Here's how the part is built. I have some questions about the finished solid (model axes, mm). Round coordinates to 2 decimals unless told otherwise and drop trailing zeros. Write each loop counter-clockwise with the first axis right and the second up, starting at its lowest first coordinate (ties: lowest second). Pieces come first, ordered by that corner, then holes. Notation, with made-up numbers: (-17, 66) - (28, 66) arc R19 cw to (28, 83) - close; hole circle Ø2 at (1, 6). An arc over 180 degrees is marked (long way). Use one line per item in the form item = value. Start each with the question number.
1. I want a section at B-B, the plane y = -1.75. List the corners of the cut face in (x, z) for me.
2. I want a section at C-C, the plane x = 230. List the corners of the cut face in (y, z) for me.
3. We'd pull the mould along Z, two halves only. Please class faces 1 (the flat face through (116, -4.5, -52)), 2 (the flat face through (-5, -9, 1)), 3 (the flat face through (-344, -4.5, -52)): +Z half, -Z half, draft (parallel to the pull), parting line (faces both ways), or undercut.
4. I want a section at A-A, the plane z = -34.5. List the corners of the cut face in (x, y) for me.
5. I want a section at D-D, the plane z = -68. List the corners of the cut face in (x, y) for me.
6. Will these pins go through, and if not, where does the flat tip stop? pin 1 (2 mm diameter, centred on x = 155.5, y = -1.5, fed in from -Z); pin 2 (2 mm diameter, centred on y = -3, z = 60, fed in from +X); pin 3 (3 mm diameter, centred on y = -2, z = -55.5, fed in from -X).
7. If I drill on line 1 along X through (y, z) = (-7.25, -6); line 2 along X through (y, z) = (-4, -78); line 3 along Z through (x, y) = (-25.5, -0.75), over which ranges is the centre line in solid material (lowest first)?
```python
from build123d import *

# Parameters (mm, degrees)
F0_W      = 740
F0_H      = 200
F1_DEPTH  = 9
F2_W      = 4.5
F2_H      = 200
F3_DEPTH  = 4.5
F4_W      = 4.5
F4_H      = 200
F5_DEPTH  = 4.5
F6_W      = 731
F6_H      = 4.5
F7_DEPTH  = 4.5
F8_W      = 731
F8_H      = 4.5
F9_DEPTH  = 4.5
F10_W     = 150
F10_H     = 95
F11_DEPTH = 25
F12_W     = 4.5
F12_H     = 40.5
F13_DEPTH = 4.5
F14_W     = 4.5
F14_H     = 40.5
F15_DEPTH = 4.5


with BuildPart() as f1:
    # F0 (on Front) → F1 (new body)
    with BuildSketch(Plane.XZ):
        Rectangle(F0_W, F0_H)
    extrude(amount=F1_DEPTH)

    # F2 (on face) → F3 (cut)
    with BuildSketch(Plane.YZ.offset(370)):
        with Locations((-2.25, 0)):
            Rectangle(F2_W, F2_H)
    extrude(amount=-F3_DEPTH, mode=Mode.SUBTRACT)

    # F4 (on face) → F5 (cut)
    with BuildSketch(Plane(origin=(-370, 0, 0), x_dir=(0, -1, 0), z_dir=(-1, 0, 0))):
        with Locations((2.25, 0)):
            Rectangle(F4_W, F4_H)
    extrude(amount=-F5_DEPTH, mode=Mode.SUBTRACT)

    # F6 (on face) → F7 (cut)
    with BuildSketch(Plane(origin=(0, 0, 0), x_dir=(-1, 0, 0), z_dir=(0, 1, 0))):
        with Locations((0, -52.75)):
            Rectangle(F6_W, F6_H)
    extrude(amount=-F7_DEPTH, mode=Mode.SUBTRACT)

    # F8 (on face) → F9 (cut)
    with BuildSketch(Plane(origin=(0, 0, 0), x_dir=(-1, 0, 0), z_dir=(0, 1, 0))):
        with Locations((0, -97.75)):
            Rectangle(F8_W, F8_H)
    extrude(amount=-F9_DEPTH, mode=Mode.SUBTRACT)

    # F10 (on face) → F11 (cut)
    with BuildSketch(Plane.XZ.offset(9)):
        with Locations((-210.5, -52.5)):
            Rectangle(F10_W, F10_H)
    extrude(amount=-F11_DEPTH, mode=Mode.SUBTRACT)

    # F12 (on face) → F13 (cut)
    with BuildSketch(Plane(origin=(0, 0, 0), x_dir=(-1, 0, 0), z_dir=(0, 1, 0))):
        with Locations((133.25, -75.25)):
            Rectangle(F12_W, F12_H)
    extrude(amount=-F13_DEPTH, mode=Mode.SUBTRACT)

    # F14 (on face) → F15 (cut)
    with BuildSketch(Plane(origin=(0, 0, 0), x_dir=(-1, 0, 0), z_dir=(0, 1, 0))):
        with Locations((287.75, -75.25)):
            Rectangle(F14_W, F14_H)
    extrude(amount=-F15_DEPTH, mode=Mode.SUBTRACT)


solid = f1.part
```
Model answer:
q1.outline = (-365.5, -95.5) - (-290, -95.5) - (-290, -55) - (-365.5, -55) - close; (-365.5, -50.5) - (-285.5, -50.5) - (-285.5, -5) - (-135.5, -5) - (-135.5, -50.5) - (365.5, -50.5) - (365.5, 100) - (-365.5, 100) - close; (-131, -95.5) - (365.5, -95.5) - (365.5, -55) - (-131, -55) - close
q2.outline = (-9, -100) - (-4.5, -100) - (-4.5, -95.5) - (0, -95.5) - (0, -55) - (-4.5, -55) - (-4.5, -50.5) - (0, -50.5) - (0, 100) - (-9, 100) - close
q3.face_1 = undercut
q3.face_2 = draft
q3.face_3 = undercut
q4.outline = (-370, -9) - (-285.5, -9) - (-285.5, 0) - (-365.5, 0) - (-365.5, -4.5) - (-370, -4.5) - close; (-135.5, -9) - (370, -9) - (370, -4.5) - (365.5, -4.5) - (365.5, 0) - (-135.5, 0) - close
q5.outline = (-370, -9) - (-285.5, -9) - (-285.5, -4.5) - (-290, -4.5) - (-290, 0) - (-365.5, 0) - (-365.5, -4.5) - (-370, -4.5) - close; (-135.5, -9) - (370, -9) - (370, -4.5) - (365.5, -4.5) - (365.5, 0) - (-131, 0) - (-131, -4.5) - (-135.5, -4.5) - close
q6.pin_1 = -95.5
q6.pin_2 = 365.5
q6.pin_3 = -365.5
q7.line_1 = -370 to -285.5, -135.5 to 370
q7.line_2 = -365.5 to -290, -131 to 365.5
q7.line_3 = -95.5 to -55, -50.5 to 100
